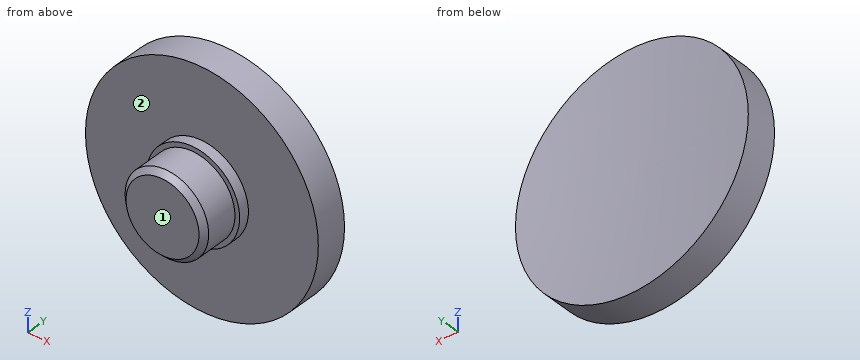
from build123d import *

# Parameters (mm, degrees)
F2_SIZE = 0.5


with BuildPart() as f1:
    # F0 (on Top) → F1 (revolve)
    with BuildSketch(Plane.XY):
        with BuildLine():
            ThreePointArc((0, 6.937257), (-5.506382, 7.093876), (-11, 7.5))
            Line((-11, 7.5), (-11, 4.5))
            Line((-11, 4.5), (-4.396255, 4.5))
            Line((-4.396255, 4.5), (-4.396255, 3.5))
            Line((-4.396255, 3.5), (-3.95, 3.5))
            Line((-3.95, 3.5), (-3.95, 0))
            Line((-3.95, 0), (0, 0))
            Line((0, 0), (0, 6.937257))
        make_face()
    revolve(axis=Axis((0, 3.75, 0), (0, 1, 0)))

    # F2
    f2_edges = [f1.edges().sort_by_distance(p)[0] for p in [
        (3.95, 0, 0),
    ]]
    chamfer(f2_edges, length=F2_SIZE)


solid = f1.part
Can you work these out from the model? Positions are in its coordinate system, mm. Face numbers are marked on the shaded views. A direction names the side the tool comes from. Round coordinates to 2 decimals unless told otherwise and drop trailing zeros. Write each loop counter-clockwise with the first axis right and the second up, starting at its lowest first coordinate (ties: lowest second). Pieces come first, ordered by that corner, then holes. Notation, with made-up numbers: (41.5, 9) -> (82.5, 9) arc R21 ccw to (82.5, 25) -> close; hole circle Ø9 at (4.25, 10). An arc over 180 degrees is marked (long way). Use one line per item in the form item = value. Start each with the question number.
Q1. I'm going to push flat-ended pins straight in: P1, Ø2, axis at x = 1, y = 2, coming from the +Z side; P2, Ø1.5, axis at y = 1, z = 4, coming from the +X side (3 decimals); P3, Ø6, axis at x = -1.5, z = -5.5, coming from the +Y side. Where does each tip first touch, or does it pass through?
Q2. Which directions (+Z, -Z, +X, -X, +Y, -Y) give clear straight access to the entire face, cutting with the end or side of a thin tool? Please do the marked faces 1 and 2.
Q3. Imagine slicing it at A-A (y = 1.75). Please give me the cut outline in (x, z).
Q4. If I drill on probe 1 along Y at (x, z) = (-4.75, 2.75); probe 2 along Z at (x, y) = (-9.5, 6.5); probe 3 along Y at (x, z) = (8.25, -6), over which ranges is the centre line in solid material (lowest first)? Write a range as [from, to].
Worked out:
q1.P1 = 3.95
q1.P2 = 2.245
q1.P3 = 7.3
q2.face_1 = +Z, -Z, +X, -X, -Y
q2.face_2 = -Y
q3.outline = circle Ø7.9 at (0, 0)
q4.probe_1 = [4.5, 7.09]
q4.probe_2 = [-5.55, 5.55]
q4.probe_3 = [4.5, 7.43]
